Verification items for this drawing (mm, ordinates from the low corner). A direction names the side the tool comes from. Round coordinates to 2 decimals unless told otherwise and drop trailing zeros. Order: outer loops, then holes, each group sorted by start corner. A loop starts at its lowest first (then second) coordinate and runs counter-clockwise, first axis right, second up. Notation, with made-up numbers: (13.5, -37) -> (47.5, -37) arc R22 cw to (47.5, -21) -> close; hole circle Ø6 at (57.25, 25). An arc over 180 degrees is marked (long way). Answer in a Markdown table with one row per item. Add a question column.
1. Material ranges on L1, parallel to Z at x = 4, y = 2.55; L2, parallel to Y at x = 13.75, z = 1.65; L3, parallel to Y at x = 8.25, z = 2.15, recorded low to high. Write a range as from..to.
2. Depth check by flat-ended pin: P1, Ø0.7, axis at x = 9, z = 2.5, coming from the +Y side. Enter the tip coordinate at first touch or a pass-through.
3. Sectioned sample at A-A, the plane z = 2.45. Record the boundary of the cut face in (x, y), then the cut area to 3 significant figures.
4. Access from +Z, -Z, +X, -X, +Y, -Y to the whole of each face (thin tool, end or side, straight path). Record for the marked faces 1 and 2.
5. Sectioned sample at C-C, the plane x = 12.5. Record the boundary of the cut face in (y, z), then the cut area to 3 significant figures.
6. Sectioned sample at B-B, the plane x = 1. Record the boundary of the cut face in (y, z).
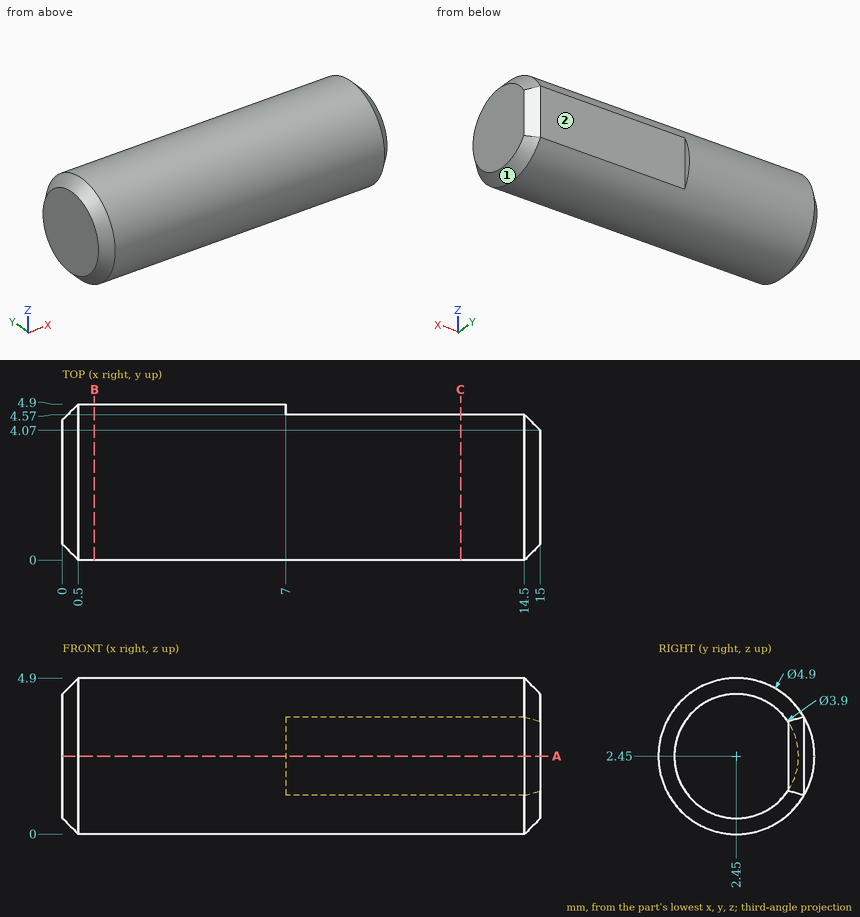
Answer key:
| question | item | result |
|---|---|---|
| 1 | L1 | z = 0..4.9 |
| 1 | L2 | y = 0.13..4.57 |
| 1 | L3 | y = 0.02..4.57 |
| 2 | P1 | stops at y = 4.57 |
| 3 | outline | (0, 0.5) -> (0.5, 0) -> (14.5, 0) -> (15, 0.5) -> (15, 4.07) -> (14.5, 4.57) -> (7, 4.57) -> (7, 4.9) -> (0.5, 4.9) -> (0, 4.4) -> close |
| 3 | area | 70.4 mm² |
| 4 | face 1 | +X |
| 4 | face 2 | +Z, -Z, +X, +Y |
| 5 | outline | (4.57, 1.22) -> (4.57, 3.68) arc R2.45 ccw (long way) to start |
| 5 | area | 18.3 mm² |
| 6 | outline | circle Ø4.9 at (2.45, 2.45) |
